Here's how the part is built. I have some questions about the finished solid (model axes, mm). A direction names the side the tool comes from. Give positions to 0.01 mm unless a question says otherwise; leave off trailing zeros. Write each loop counter-clockwise with the first axis right and the second up, starting at its lowest first coordinate (ties: lowest second). Pieces come first, ordered by that corner, then holes. Notation, with made-up numbers: (43.5, -26) -> (49.5, -26) arc R10 ccw to (49.5, -9) -> close; hole circle Ø4 at (35, 63.5). An arc over 180 degrees is marked (long way). Use CSV: the item, a comma, the result in double quotes. Start each with the question number.
(1) If we mould it in two halves opening along Y, with no side actions, what happens to faces 1 (the flat face through (-1, 6, -5)), 2 (the flat face through (-1, -15, -1)), 3 (the flat face through (52.63, -11.394, 18.479))? For each: pulls with the +Y half, pulls with the -Y half, needs draft (parallel to the pull), parting line crosses it, or undercut.
(2) For pin 1 Ø8 at (x, y) = (32, 0.5) entering from +Z; pin 2 Ø3 at (x, y) = (-55.5, 10) entering from +Z; pin 3 Ø5 at (x, z) = (-20, 15.5) entering from -Y, each with a flat end and sliding along its axis, tell me the tip position at first contact or that it passes through.
(3) Suppose I cut it at C-C on z = 7.25. Give the number of separate pieces and of enclosed holes in the cut face, plus the area to 3 significant figures.
(4) I need wall thicknesses on L1, parallel to Y at x = 55, z = 6.75; L2, parallel to X at y = -4, z = 18; L3, parallel to Y at x = 52, z = 18.25. Which ranges of each line are inside material? Lowest first, please. Write a range as [from, to].
(5) Suppose I cut it at B-B on y = -0.5. List the corners of the cut face in (x, z) for me.
(6) Suppose I cut it at D-D on x = -43. List the corners of the cut face in (y, z) for me, plus the area to 3 significant figures.
(7) Which directions (+Z, -Z, +X, -X, +Y, -Y) give clear straight access to the entire face, cutting with the end or side of a thin tool? Please do faces 4 (the flat face through (-39, 5, 15)), 5 (the flat face through (-26.5, 5, 8)), 6 (the cylindrical face through (56.386, -10.575, 5.846)).
(8) Suppose I cut it at A-A on x = 55. List the corners of the cut face in (y, z) for me.
from build123d import *

# Parameters (mm, degrees)
ESQUISSE1_W             = 120
ESQUISSE1_H             = 30
ESQUISSE1_R             = 1.5
BOSS_EXTRU_1_DEPTH      = 5
BOSS_EXTRU_2_DEPTH      = 20
BOSS_EXTRU_3_DEPTH      = 10
ESQUISSE1_6_R           = 1.5
BOSS_EXTRU_4_DEPTH      = 17
ESQUISSE2_R             = 1.4
ENL_V_MAT_EXTRU_1_DEPTH = 26
BOSS_EXTRU_5_DEPTH      = 10
ESQUISSE4_W             = 120
ESQUISSE4_H             = 25
BOSS_EXTRU_6_DEPTH      = 3


with BuildPart() as part:
    # Esquisse1 → Boss.-Extru.1 (new body)
    with BuildSketch(Plane.XY):
        Rectangle(ESQUISSE1_W, ESQUISSE1_H)
        with Locations((-55, 10)):
            Circle(ESQUISSE1_R, mode=Mode.SUBTRACT)
        with Locations((-55, -10)):
            Circle(ESQUISSE1_R, mode=Mode.SUBTRACT)
        with Locations((55, -10)):
            Circle(ESQUISSE1_R, mode=Mode.SUBTRACT)
        with Locations((55, 10)):
            Circle(ESQUISSE1_R, mode=Mode.SUBTRACT)
    extrude(amount=-BOSS_EXTRU_1_DEPTH)

    # Esquisse1<4> → Boss.-Extru.2 (add)
    with BuildSketch(Plane.XY):
        Polygon((-26.5, 15), (-60, 15), (-60, -15), (-26.5, -15), (-26.5, -5), (-50.7, -5), (-50.7, -3), (-53.5, -3), (-53.5, 3), (-50.7, 3), (-50.7, 5), (-26.5, 5), align=None)
        Polygon((-53.41228676, 12.75), (-51.824573519, 10), (-53.41228676, 7.25), (-56.58771324, 7.25), (-58.175426481, 10), (-56.58771324, 12.75), align=None, mode=Mode.SUBTRACT)
        Polygon((-53.41228676, -7.25), (-51.824573519, -10), (-53.41228676, -12.75), (-56.58771324, -12.75), (-58.175426481, -10), (-56.58771324, -7.25), align=None, mode=Mode.SUBTRACT)
        Polygon((60, 15), (26.5, 15), (26.5, 5), (50.7, 5), (50.7, 3), (53.5, 3), (53.5, -3), (50.7, -3), (50.7, -5), (26.5, -5), (26.5, -15), (60, -15), align=None)
        Polygon((56.58771324, 7.25), (53.41228676, 7.25), (51.824573519, 10), (53.41228676, 12.75), (56.58771324, 12.75), (58.175426481, 10), align=None, mode=Mode.SUBTRACT)
        Polygon((56.58771324, -7.25), (58.175426481, -10), (56.58771324, -12.75), (53.41228676, -12.75), (51.824573519, -10), (53.41228676, -7.25), align=None, mode=Mode.SUBTRACT)
    extrude(amount=BOSS_EXTRU_2_DEPTH)

    # Esquisse1<5> → Boss.-Extru.3 (add)
    with BuildSketch(Plane.XY):
        Polygon((-26.5, -5), (-26.5, 5), (-50.7, 5), (-50.7, 3), (-53.5, 3), (-53.5, -3), (-50.7, -3), (-50.7, -5), align=None)
        Polygon((50.7, 5), (26.5, 5), (26.5, -5), (50.7, -5), (50.7, -3), (53.5, -3), (53.5, 3), (50.7, 3), align=None)
    extrude(amount=BOSS_EXTRU_3_DEPTH)

    # Esquisse1<6> → Boss.-Extru.4 (add)
    with BuildSketch(Plane.XY):
        Polygon((51.824573519, 10), (53.41228676, 12.75), (56.58771324, 12.75), (58.175426481, 10), (56.58771324, 7.25), (53.41228676, 7.25), align=None)
        with Locations((55, 10)):
            Circle(ESQUISSE1_6_R, mode=Mode.SUBTRACT)
        Polygon((56.58771324, -7.25), (53.41228676, -7.25), (51.824573519, -10), (53.41228676, -12.75), (56.58771324, -12.75), (58.175426481, -10), align=None)
        with Locations((55, -10)):
            Circle(ESQUISSE1_6_R, mode=Mode.SUBTRACT)
        Polygon((-56.58771324, 7.25), (-53.41228676, 7.25), (-51.824573519, 10), (-53.41228676, 12.75), (-56.58771324, 12.75), (-58.175426481, 10), align=None)
        with Locations((-55, 10)):
            Circle(ESQUISSE1_6_R, mode=Mode.SUBTRACT)
        Polygon((-51.824573519, -10), (-53.41228676, -12.75), (-56.58771324, -12.75), (-58.175426481, -10), (-56.58771324, -7.25), (-53.41228676, -7.25), align=None)
        with Locations((-55, -10)):
            Circle(ESQUISSE1_6_R, mode=Mode.SUBTRACT)
    extrude(amount=BOSS_EXTRU_4_DEPTH)

    # Esquisse2 → Enlèv. mat.-Extru.1 (cut, through all)
    with BuildSketch(Plane.XY.offset(20)):
        with Locations((-38.6, 10)):
            Circle(ESQUISSE2_R)
        with Locations((-37.6, -10)):
            Circle(ESQUISSE2_R)
        with Locations((38.6, 10)):
            Circle(ESQUISSE2_R)
        with Locations((37.6, -10)):
            Circle(ESQUISSE2_R)
    extrude(amount=-ENL_V_MAT_EXTRU_1_DEPTH, mode=Mode.SUBTRACT)

    # Esquisse3 → Boss.-Extru.5 (add)
    with BuildSketch(Plane(origin=(0, 15, 0), x_dir=(1, 0, 0), z_dir=(0, 1, 0))):
        Polygon((-60, -20), (-60, 5), (60, 5), (60, -20), (26.5, -20), (26.5, 0), (-26.5, 0), (-26.5, -20), align=None)
    extrude(amount=BOSS_EXTRU_5_DEPTH)

    # Esquisse4 → Boss.-Extru.6 (add)
    with BuildSketch(Plane(origin=(0, 25, 0), x_dir=(1, 0, 0), z_dir=(0, 1, 0))):
        with Locations((0, -7.5)):
            Rectangle(ESQUISSE4_W, ESQUISSE4_H)
    extrude(amount=BOSS_EXTRU_6_DEPTH)


solid = part.part
Geometry says:
1,face 1,"needs draft"
1,face 2,"pulls with the -Y half"
1,face 3,"undercut"
2,pin 1,"z = 10"
2,pin 2,"z = 17"
2,pin 3,"y = 25"
3,separate pieces,"1"
3,enclosed holes,"8"
3,area,"2,990 mm²"
4,L1,"[-15, -11.5], [-8.5, 8.5], [11.5, 28]"
4,L2,"[-60, -50.7], [50.7, 60]"
4,L3,"[-15, -10.3], [-9.7, -3], [3, 9.7], [10.3, 28]"
5,outline,"(-60, -5) -> (60, -5) -> (60, 20) -> (53.5, 20) -> (53.5, 10) -> (26.5, 10) -> (26.5, 0) -> (-26.5, 0) -> (-26.5, 10) -> (-53.5, 10) -> (-53.5, 20) -> (-60, 20) -> close"
6,outline,"(-15, -5) -> (28, -5) -> (28, 20) -> (5, 20) -> (5, 10) -> (-5, 10) -> (-5, 20) -> (-15, 20) -> close"
6,area,"975 mm²"
7,face 4,"+Z"
7,face 5,"+Z, -Y"
7,face 6,"+Z, -Z"
8,outline,"(-15, -5) -> (-11.5, -5) -> (-11.5, 17) -> (-12.75, 17) -> (-12.75, 20) -> (-15, 20) -> close; (-8.5, -5) -> (8.5, -5) -> (8.5, 17) -> (7.25, 17) -> (7.25, 20) -> (-7.25, 20) -> (-7.25, 17) -> (-8.5, 17) -> close; (11.5, -5) -> (28, -5) -> (28, 20) -> (12.75, 20) -> (12.75, 17) -> (11.5, 17) -> close"
